Model file for the job. Use its own axes, mm. Face numbers are marked on the shaded views. A direction names the side the tool comes from. Coordinates: 2 decimals unless noted, no trailing zeros. Order: outer loops, then holes, each group sorted by start corner. A loop starts at its lowest first (then second) coordinate and runs counter-clockwise, first axis right, second up. Notation, with made-up numbers: (33.5, 52.25) - (42.5, 52.25) arc R26 ccw to (42.5, 69.25) - close; hole circle Ø10 at (5, -1). An arc over 180 degrees is marked (long way). Put each result on its own line as item: value. Start each with the question number.
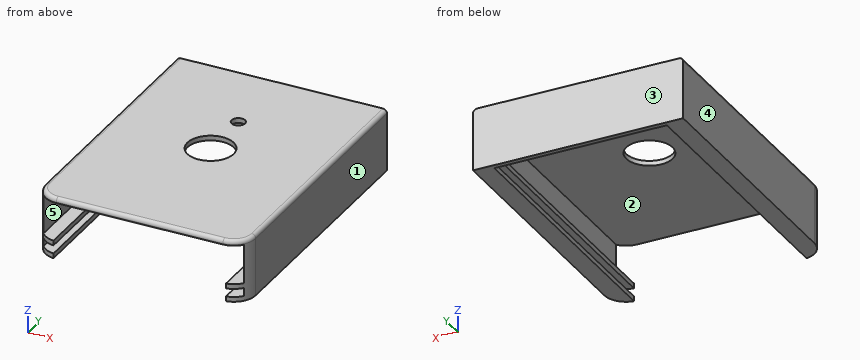
Autodesk Fusion 360 part; units mm, degrees
sketch "Sketch1" plane through (0, 0, 0) normal (0, 0, 1) x (1, 0, 0)
  line L0 (0, 0) -> (73.6, 0)
  line L1 (73.6, 0) -> (73.6, 100.6)
  line L2 (73.6, 100.6) -> (0, 100.6)
  line L3 (0, 100.6) -> (0, 0)
  line L4 (5.1, 0) -> (68.5, 0)
  line L5 (68.5, 0) -> (68.5, 100.6)
  line L6 (68.5, 100.6) -> (5.1, 100.6)
  line L7 (5.1, 100.6) -> (5.1, 0)
  line L8 (-1.8, 0) -> (75.4, 0)
  line L9 (75.4, 0) -> (75.4, 100.6)
  line L10 (75.4, 100.6) -> (-1.8, 100.6)
  line L11 (-1.8, 100.6) -> (-1.8, 0)
  dimension "d1" = 73.6
  dimension "d2" = 100.6
  dimension "d3" = 63.4
  dimension "d4" = 5.1
  dimension "d6" = 1.8
  dimension "d7" = 1.8
extrude "Extrude1" add sketch "Sketch1" along normal blind 1.8 contours L0 L2 L3 L7 L8 L10 | L3 L8 L10 L11 | L0 L1 L2 L5 L8 L10 | L1 L8 L9 L10 makes body 1 at (70.8, 33.5333, 0) makes body 2 at (0.5, 67.0667, 0)
extrude "Extrude2" add sketch "Sketch1" along normal blind 4.8 separate body contours L3 L8 L10 L11 | L1 L8 L9 L10 makes body 3 at (-1.8, 67.0667, 1.6) makes body 4 at (75.4, 33.5333, 1.6)
extrude "Extrude3" add sketch "Sketch1" along normal blind 1.8 from surface at 4.8 separate body contours L0 L2 L3 L7 L8 L10 | L3 L8 L10 L11 | L0 L1 L2 L5 L8 L10 | L1 L8 L9 L10 makes body 5 at (70.8, 33.5333, 4.8) makes body 6 at (0.5, 67.0667, 4.8)
extrude "Extrude4" add sketch "Sketch1" along normal blind 16 from surface at 5 separate body contours L3 L8 L10 L11 | L1 L8 L9 L10 makes body 7 at (75.4, 33.5333, 10.3333) makes body 8 at (-1.8, 67.0667, 10.3333)
extrude "Extrude5" add sketch "Sketch1" along normal blind 1.8 from surface at 21 separate body makes body 9
sketch "Sketch2" plane through (0, 100.6, 0) normal (0, 1, 0) x (-1, 0, 0)
  line L0 (-75.4, 21) -> (1.8, 21)
  line L1 (1.8, 21) -> (1.8, 22.8)
  line L2 (1.8, 22.8) -> (-75.4, 22.8)
  line L3 (-75.4, 22.8) -> (-75.4, 21)
  line L4 (-75.4, 0) -> (1.8, 0)
  line L5 (1.8, 0) -> (1.8, 22.8)
  line L6 (1.8, 22.8) -> (-75.4, 22.8)
  line L7 (-75.4, 22.8) -> (-75.4, 0)
  line L8 (1.8, 5) -> (1.8, 21)
  line L9 (-75.4, 5) -> (-75.4, 21)
  line L10 (-75.4, 0) -> (1.8, 0)
extrude "Extrude6" add sketch "Sketch2" along normal blind 1.8 bodies 1 2 3 4 5 6 7 8 9
fillet "Fillet1" radius 8 2 edges at (-1.8, 0, 11.4) (75.4, 0, 11.4) on bodies 1
fillet "Fillet2" radius 1.5 5 edges at (-1.8, 55.2, 22.8) (0.5431, 2.3431, 22.8) (36.8, 0, 22.8) (73.0569, 2.3431, 22.8) (75.4, 55.2, 22.8) on bodies 1
sketch "Sketch3" plane through (0, 0, 22.8) normal (0, 0, 1) x (-1, 0, 0)
  line L0 (0.3, -102.4) -> (0.3, -8)
  arc A0 (0.3, -8) -> (-6.2, -1.5) centre (-6.2, -8) ccw
  line L1 (-6.2, -1.5) -> (-67.4, -1.5)
  arc A1 (-67.4, -1.5) -> (-73.9, -8) centre (-67.4, -8) ccw
  line L2 (-73.9, -8) -> (-73.9, -102.4)
  line L3 (-73.9, -102.4) -> (0.3, -102.4)
  line L4 (0.3, -102.4) -> (-71.9962, -3.4038) construction
  circle A2 centre (-35.8481, -52.9019) radius 8.5
  line L5 (-35.8481, -72.9019) -> (-35.8481, -52.9019)
  circle A3 centre (-35.8481, -72.9019) radius 2.5
  dimension "d26" = 17
  dimension "d27" = 20
  dimension "d28" = 5
extrude "Extrude7" cut sketch "Sketch3" against normal blind 1.8 contours A2 | A3 bodies 1
equation "d4 = ( 10.2 / 2 ) * 1 mm"
equation "d6 = Linear Dimension-6"
equation "d7 = Linear Dimension-7"
equation "d10 = t + 3 mm"
equation "d12 = t + 3 mm"
equation "ra = 8 mm"
equation "d16 = 2 mm + 3 mm"
equation "d19 = 19 mm + 2 mm"
equation "d24 = ra"
Item 1: Slice it at D-D, the plane x = 23.5. Give the cut face in (y, z), plus the area to 3 significant figures.
Item 2: Slice it at B-B, the plane y = 27. Give the cut face in (x, z).
Item 3: Wall check: line 1 along Z through (x, y) = (70.5, 22); line 2 along X through (y, z) = (94.5, 16.75); line 3 along X through (y, z) = (14.5, 1). Give the ranges that are in metal, low to high.
Item 4: 3-axis set-ups, long thin cutter, end or side, ignore diameter. For the marked faces 1 and 2: which of +Z, -Z, +X, -X, +Y, -Y reach the whole face in a straight line?
Item 5: Pull direction X, two halves, no side cores. Call the marked faces 3, 4 and 5: pulls with the +X half, pulls with the -X half, needs draft (parallel to the pull), parting line crosses it, or undercut.
Item 6: Slice it at A-A, the plane x = 40.5. Give the cut face in (y, z), plus the area to 3 significant figures.
Item 7: Slice it at C-C, the plane z = 11. Give the cut face in (x, y), plus the area to 3 significant figures.
Item 8: Flat gauge pin, fed straight in: pin 1 Ø1.5 at (x, z) = (8.5, 3) entering from -Y. Where does the tip first touch, or does it go through?
Here are the results:
1. outline: (0, 21) - (100.6, 21) - (100.6, 0) - (102.4, 0) - (102.4, 22.8) - (1.5, 22.8) arc R1.5 ccw to (0, 21.3) - close
1. area: 222 mm^2
2. outline: (-1.8, 0) - (5.1, 0) - (5.1, 1.8) - (0, 1.8) - (0, 4.8) - (5.1, 4.8) - (5.1, 6.6) - (0, 6.6) - (0, 21) - (73.6, 21) - (73.6, 6.6) - (68.5, 6.6) - (68.5, 4.8) - (73.6, 4.8) - (73.6, 1.8) - (68.5, 1.8) - (68.5, 0) - (75.4, 0) - (75.4, 21.3) arc R1.5 ccw to (73.9, 22.8) - (-0.3, 22.8) arc R1.5 ccw to (-1.8, 21.3) - close
3. line 1: z = 0 to 1.8, 4.8 to 6.6, 21 to 22.8
3. line 2: x = -1.8 to 0, 73.6 to 75.4
3. line 3: x = -1.8 to 5.1, 68.5 to 75.4
4. face 1: +Z, -Z, +X, +Y, -Y
4. face 2: -Y
5. face 3: needs draft
5. face 4: pulls with the -X half
5. face 5: undercut
6. outline: (0, 21) - (45.79, 21) - (45.79, 22.8) - (1.5, 22.8) arc R1.5 ccw to (0, 21.3) - close; (60.02, 21) - (100.6, 21) - (100.6, 0) - (102.4, 0) - (102.4, 22.8) - (60.02, 22.8) - close
6. area: 196 mm^2
7. outline: (-1.8, 8) arc R8 ccw to (0, 2.94) - (0, 100.6) - (73.6, 100.6) - (73.6, 2.94) arc R8 ccw to (75.4, 8) - (75.4, 102.4) - (-1.8, 102.4) - close
7. area: 485 mm^2
8. pin 1: stops at y = 100.6
